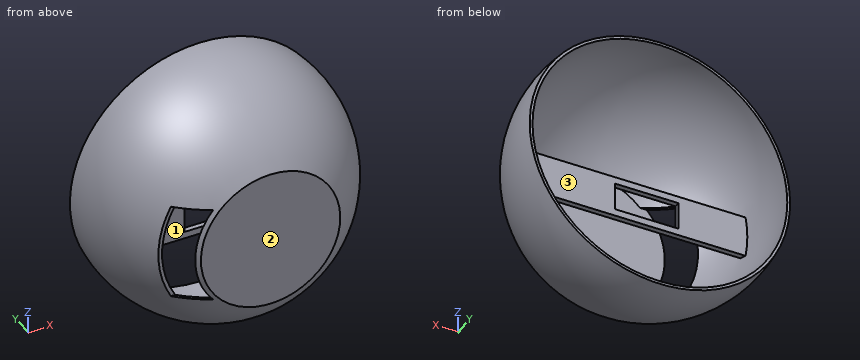
from build123d import *

# Parameters (mm, degrees)
SHELL_1_T            = -1
EXTRUDE_1_REACH      = 80.75
EXTRUDE_1_END_RADIUS = 46.75
SKETCH_2_W           = 15
SKETCH_2_H           = 2
EXTRUDE_2_REACH      = 80.75
SKETCH_4_W           = 15
SKETCH_4_H           = 2
SKETCH_5_W           = 23
SKETCH_5_H           = 10
CUT_EXTRUDE_1_DEPTH  = 10
SKETCH_6_W           = 35
SKETCH_6_H           = 8
CUT_EXTRUDE_2_DEPTH  = 47


with BuildPart() as part:
    # 草图1 → 旋转1 (revolve)
    with BuildSketch(Plane(origin=(0, 0, 0), x_dir=(0, 0, -1), z_dir=(1, 0, 0))):
        with BuildLine():
            Line((-47.200739576, 7.221681487), (0, 7.221681487))
            Line((0, 7.221681487), (0, -40.513710474))
            Line((0, -40.513710474), (-25.272549608, -40.513710474))
            ThreePointArc((-25.272549608, -40.513710474), (-43.390797673, -19.932415241), (-47.200739576, 7.221681487))
        make_face()
    revolve(axis=Axis((0, 7.221681487, 0), (0, -1, 0)))

    # 抽壳1
    shell_1_openings = [part.faces().sort_by_distance(p)[0] for p in [
        (0, 7.221681487, 0),
    ]]
    offset(amount=SHELL_1_T, openings=shell_1_openings, kind=Kind.INTERSECTION)

    # 凸台-拉伸1: up to this sphere (the profile starts inside it)
    extrude_1_end = Location((0, 0, 0)) * Sphere(EXTRUDE_1_END_RADIUS, mode=Mode.PRIVATE)
    # 草图2 → 凸台-拉伸1 (add, up to the surface)
    with BuildSketch(Plane(origin=(0, 0, 0), x_dir=(0, 0, -1), z_dir=(1, 0, 0)), mode=Mode.PRIVATE) as extrude_1_sk1:
        with Locations((0, -16.778318513)):
            Rectangle(SKETCH_2_W, SKETCH_2_H)
    extrude_1_tool1 = extrude(extrude_1_sk1.sketch, amount=EXTRUDE_1_REACH, mode=Mode.PRIVATE) & extrude_1_end
    add(extrude_1_tool1.solids().sort_by_distance((0, -16.778319, 0))[0])

    # 草图4 → 凸台-拉伸2 (add, up to next)
    with BuildSketch(Plane(origin=(0, 0, 0), x_dir=(0, 0, -1), z_dir=(1, 0, 0)), mode=Mode.PRIVATE) as extrude_2_sk1:
        with Locations((0, -16.778318513)):
            Rectangle(SKETCH_4_W, SKETCH_4_H)
    extrude_2_tool1 = extrude(extrude_2_sk1.sketch, amount=-EXTRUDE_2_REACH, mode=Mode.PRIVATE) - part.part
    add(extrude_2_tool1.solids().sort_by_distance((0, -16.778319, 0))[0])

    # 草图5 → 切除-拉伸1 (cut)
    with BuildSketch(Plane(origin=(0, -15.778318513, 0), x_dir=(1, 0, 0), z_dir=(0, 1, 0))):
        with Locations((-7.5, 0)):
            Rectangle(SKETCH_5_W, SKETCH_5_H)
    extrude(amount=-CUT_EXTRUDE_1_DEPTH, mode=Mode.SUBTRACT)

    # 草图6 → 切除-拉伸2 (cut)
    with BuildSketch(Plane(origin=(0, 0, 0), x_dir=(0, 0, -1), z_dir=(1, 0, 0))):
        with Locations((0, -35.513710474)):
            Rectangle(SKETCH_6_W, SKETCH_6_H)
    extrude(amount=-CUT_EXTRUDE_2_DEPTH, mode=Mode.SUBTRACT)


solid = part.part
Could you check a few things on this model? Use its own coordinates, in mm. Face numbers are marked on the shaded views. Give positions to 0.01 mm unless a question says otherwise; leave off trailing zeros. Write each loop counter-clockwise with the first axis right and the second up, starting at its lowest first coordinate (ties: lowest second). Pieces come first, ordered by that corner, then holes. Notation, with made-up numbers: (28.5, 47) -> (66.5, 47) arc R13 cw to (66.5, 72) -> close; hole circle Ø8 at (59, 68). An arc over 180 degrees is marked (long way). Answer as a JSON object with one key per item and string values.
Q1. Will these pins go through, and if not, where does the flat tip stop? pin 1 Ø12 at (x, z) = (-10.5, 3) entering from +Y; pin 2 Ø5 at (x, y) = (-15.5, -11) entering from +Z; pin 3 Ø8 at (x, y) = (30.5, -26.5) entering from -Z.
Taken from the geometry:
{"pin 1": "stops at y = -15.78", "pin 2": "stops at z = 44.81", "pin 3": "stops at z = -30.9"}
Q2. We'd pull the mould along Y, two halves only. Please class the marked faces 1, 2 and 3: released by +Y, released by -Y, zero draft, split by the parting line, or undercut.
Taken from the geometry:
{"face 1": "undercut", "face 2": "released by -Y", "face 3": "released by +Y"}
Q3. Suppose I cut it at A-A on x = -33. Write out the boundary of the cut face in (y, z), then the cut area to 3 significant figures.
Taken from the geometry:
{"outline": "(-31.51, -14.07) arc R34.51 ccw to (7.22, -33.75) -> (7.22, -32.32) arc R33.11 cw to (-31.51, -10.17) -> close; (-31.51, 10.17) arc R33.11 cw to (7.22, 32.32) -> (7.22, 33.75) arc R34.51 ccw to (-31.51, 14.07) -> close; (-17.78, -7.5) -> (-15.78, -7.5) -> (-15.78, 7.5) -> (-17.78, 7.5) -> close", "area": "164 mm²"}
Q4. Suppose I cut it at B-B on z = 2. Write out the boundary of the cut face in (x, y).
Taken from the geometry:
{"outline": "(-47.16, 7.22) arc R47.71 ccw to (-35.82, -31.51) -> (-34.47, -31.51) arc R46.71 cw to (-43.19, -17.78) -> (-19, -17.78) -> (-19, -15.78) -> (-43.96, -15.78) arc R46.71 cw to (-46.15, 7.22) -> close; (-26.73, -39.51) arc R47.71 ccw to (-25.19, -40.51) -> (25.19, -40.51) arc R47.71 ccw to (47.16, 7.22) -> (46.15, 7.22) arc R46.71 cw to (43.96, -15.78) -> (4, -15.78) -> (4, -17.78) -> (43.19, -17.78) arc R46.71 cw to (24.9, -39.51) -> close"}
Q5. Suppose I cut it at D-D on y = -12.5. Write out the boundary of the cut face in (x, z).
Taken from the geometry:
{"outline": "circle Ø92.17 at (0, 0); hole circle Ø90.1 at (0, 0)"}
Q6. Suppose I cut it at C-C on x = 8. Write out the boundary of the cut face in (y, z), then the cut area to 3 significant figures.
Taken from the geometry:
{"outline": "(-40.51, -23.97) arc R47.08 ccw to (7.22, -46.52) -> (7.22, -45.49) arc R46.06 cw to (-39.51, -23.67) -> (-39.51, 23.67) arc R46.06 cw to (7.22, 45.49) -> (7.22, 46.52) arc R47.08 ccw to (-40.51, 23.97) -> close; (-17.78, -7.5) -> (-15.78, -7.5) -> (-15.78, 7.5) -> (-17.78, 7.5) -> close", "area": "190 mm²"}
Q7. Please list where these lines run through material, in increasing order: L1, parallel to X at y = -10, z = -35.5; L2, parallel to Y at x = 0, z = 4; L3, parallel to Z at x = 17, y = -9.5.
Taken from the geometry:
{"L1": "x = -30.33 to -28.73, 28.73 to 30.33", "L2": "y = -40.51 to -39.51", "L3": "z = -43.6 to -42.5, 42.5 to 43.6"}
